Geometry: see drawing. Coordinates: mm, zero at the bounding-box minimum. A direction names the side the tool comes from. Give positions to 0.01 mm unless a question says otherwise; leave off trailing zeros. Write each loop counter-clockwise with the first axis right and the second up, starting at its lowest first coordinate (ties: lowest second). Pieces come first, ordered by that corner, then holes. Notation, with made-up numbers: (-7, 5.5) - (41, 5.5) arc R8 ccw to (41, 13.5) - close; hole circle Ø6 at (-13.5, 6). An arc over 180 degrees is marked (long way). One line per question, with ' | ' between items. Start each with the question number.
(1) Pin query (flat end, axial travel): pin 1 (2 mm diameter, centred on y = 121.5, z = 2, fed in from -X); pin 2 (20 mm diameter, centred on x = 76.2, y = 122.16, fed in from -Z); pin 3 (12 mm diameter, centred on x = 81.5, y = 83.5, fed in from +Z); pin 4 (5 mm diameter, centred on x = 126, z = 9.5, fed in from +Y). Return the tip coordinate at first contact, or that it passes through.
(2) Section B-B, the plane y = 119. Return loops of the section in (x, z) (1 decimal), plus the area to 3 significant figures.
(3) Section D-D, the plane y = 83. Return loops of the section in (x, z) (1 decimal).
(4) Section C-C, the plane z = 6. Return loops of the section in (x, y), plus the area to 3 significant figures.
(5) Access query for the marked faces 4 and 5. Directions: +Z, -Z, +X, -X, +Y, -Y. A direction counts if a zero-diameter tool reaches every point of the face in a straight line with its end or side. Return the directions, or none.
(6) Section A-A, the plane x = 76.2. Return loops of the section in (y, z), plus the area to 3 significant figures.
(7) Draft query along X for the marked faces 1, 2 and 3. Return one class per face: +X half, -X half, draft (parallel to the pull), parting line (faces both ways), or undercut.
(8) Ray query, line 1 (Y direction, x = 76.2, z = 11); line 2 (X direction, y = 82.5, z = 8.25) (1 decimal); line 3 (X direction, y = 32, z = 8.75). Return the intervals inside material, ascending. Write a range as [from, to].
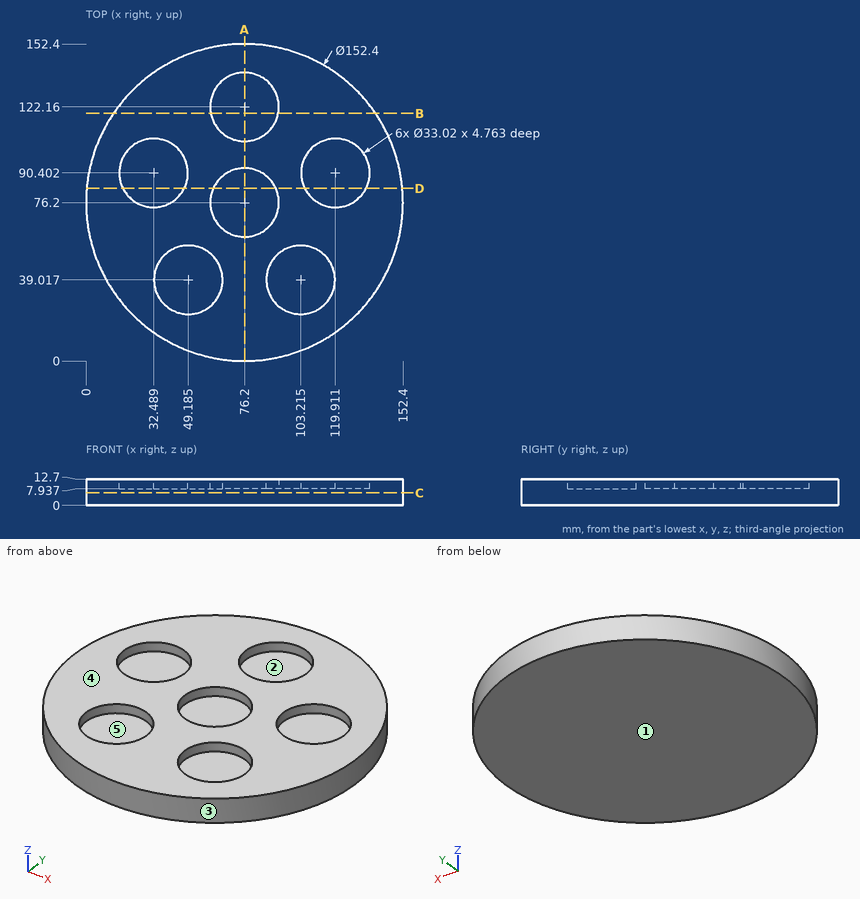
Check sheet entries:
1) pin 1: x = 14.2 | pin 2: z = 0 | pin 3: z = 7.94 | pin 4: y = 135.94
2) outline: (13.2, 0) - (139.2, 0) - (139.2, 12.7) - (92.4, 12.7) - (92.4, 7.9) - (60, 7.9) - (60, 12.7) - (13.2, 12.7) - close | area: 1,450 mm²
3) outline: (0.3, 0) - (152.1, 0) - (152.1, 12.7) - (134.7, 12.7) - (134.7, 7.9) - (105.2, 7.9) - (105.2, 12.7) - (91.2, 12.7) - (91.2, 7.9) - (61.2, 7.9) - (61.2, 12.7) - (47.2, 12.7) - (47.2, 7.9) - (17.7, 7.9) - (17.7, 12.7) - (0.3, 12.7) - close
4) outline: circle Ø152.4 at (76.2, 76.2) | area: 18,200 mm²
5) face 4: +Z, +X, -X, +Y, -Y | face 5: +Z
6) outline: (0, 0) - (152.4, 0) - (152.4, 12.7) - (138.67, 12.7) - (138.67, 7.94) - (105.65, 7.94) - (105.65, 12.7) - (92.71, 12.7) - (92.71, 7.94) - (59.69, 7.94) - (59.69, 12.7) - (0, 12.7) - close | area: 1,620 mm²
7) face 1: draft | face 2: undercut | face 3: parting line
8) line 1: [0, 59.69], [92.71, 105.65], [138.67, 152.4] | line 2: [0.3, 18], [47, 60.9], [91.5, 105.4], [134.4, 152.1] | line 3: [14.13, 34.24], [64.13, 88.27], [118.16, 138.27]
